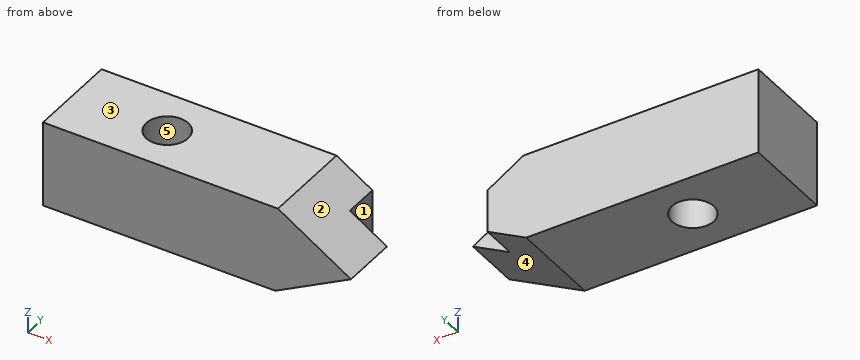
from build123d import *

# Parameters (mm, degrees)
EXTRUDE_1_DEPTH     = 26
SKETCH_3_R          = 5.915746271
SKETCH_3_W          = 24.366628961
SKETCH_3_H          = 13.595872682
CUT_EXTRUDE_2_DEPTH = 46


with BuildPart() as part:
    # 스케치2 → 보스-돌출1 (new body)
    with BuildSketch(Plane(origin=(0, 0, 0), x_dir=(1, 0, 0), z_dir=(0, 1, 0))):
        Polygon((-30.145598194, 0), (-30.145598194, 24.253001272), (35.467738861, 24.253001272), (56.854401806, 12.789785553), (36.233634312, 0), align=None)
    extrude(amount=EXTRUDE_1_DEPTH)

    # 스케치3 → 컷-돌출2 (cut)
    with BuildSketch(Plane.XY):
        with Locations((-3.33144194, 13)):
            Circle(SKETCH_3_R)
        with Locations((58.556264228, 22.797936341)):
            Rectangle(SKETCH_3_W, SKETCH_3_H)
    extrude(amount=-CUT_EXTRUDE_2_DEPTH, mode=Mode.SUBTRACT)


solid = part.part
Here's how the part is built. I have some questions about the finished solid (model axes, mm). Face numbers are marked on the shaded views. A direction names the side the tool comes from. Round coordinates to 2 decimals unless told otherwise and drop trailing zeros. Loops run counter-clockwise (first coordinate to the right, second up) from the corner with the lowest first, then second, coordinate; pieces in that order, holes last. Notation, with made-up numbers: M -4,79.25 L 1,79.25 A28 ccw 1,97.25 Z; hole C 20,-9.5 d5. An arc over 180 degrees is marked long. Write each question's results on one line, items separated by ' | '. Start each with the question number.
(1) I want a section at C-C (y = 3). Please give me the cut outline in (x, z), then the cut area to 3 significant figures.
(2) On a 3-axis mill with a long thin cutter (end or side, diameter ignored), from which of +Z, -Z, +X, -X, +Y, -Y can I reach the whole of each face in a straight line? I mean the marked faces 1 and 2. Say none if no direction works.
(3) I want a section at D-D (y = 21). Please give me the cut outline in (x, z), then the cut area to 3 significant figures.
(4) If I drill on probe 1 along X at (y, z) = (16.75, -5); probe 2 along X at (y, z) = (14, -15.75); probe 3 along X at (y, z) = (3.5, -4.25), over which ranges is the centre line in solid material (lowest first)? Write a range as from..to.
(5) I want a section at B-B (z = -21). Please give me the cut outline in (x, y), then the cut area to 3 significant figures.
(6) Will these pins go through, and if not, where does the flat tip stop? P1, Ø1, axis at y = 2.5, z = -19, coming from the +X side; P2, Ø3, axis at y = 19.5, z = -15, coming from the +X side; P3, Ø11.5, axis at x = 52.5, z = -13.5, coming from the +Y side.
(7) Thinking about a two-plate mould opening in X: for the marked faces 3, 4 and 5, which applies, pulls with the +X half, pulls with the -X half, needs draft (parallel to the pull), parting line crosses it, or undercut?
(8) I want a section at A-A (y = 13). Please give me the cut outline in (x, z).
Solved:
1) outline: M -30.15,-24.25 L 35.47,-24.25 L 56.85,-12.79 L 36.23,0 L -30.15,0 Z | area: 1,860 mm²
2) face 1: +Z, -Z, +X, +Y | face 2: +Z, +X, +Y, -Y
3) outline: M -30.15,-24.25 L 35.47,-24.25 L 46.37,-18.41 L 46.37,-6.29 L 36.23,0 L -30.15,0 Z | area: 1,790 mm²
4) probe 1: x = -30.15..-7.91, 1.24..44.3 | probe 2: x = -30.15..-9.16, 2.5..51.33 | probe 3: x = -30.15..43.09
5) outline: M -30.15,0 L 41.54,0 L 41.54,26 L -30.15,26 Z; hole C -3.33,13 d11.83 | area: 1,750 mm²
6) P1: stops at x = 46.2 | P2: stops at x = 46.37 | P3: stops at y = 16
7) face 3: needs draft | face 4: pulls with the +X half | face 5: undercut
8) outline: M -30.15,-24.25 L -9.25,-24.25 L -9.25,0 L -30.15,0 Z; M 2.58,-24.25 L 35.47,-24.25 L 56.85,-12.79 L 36.23,0 L 2.58,0 Z
